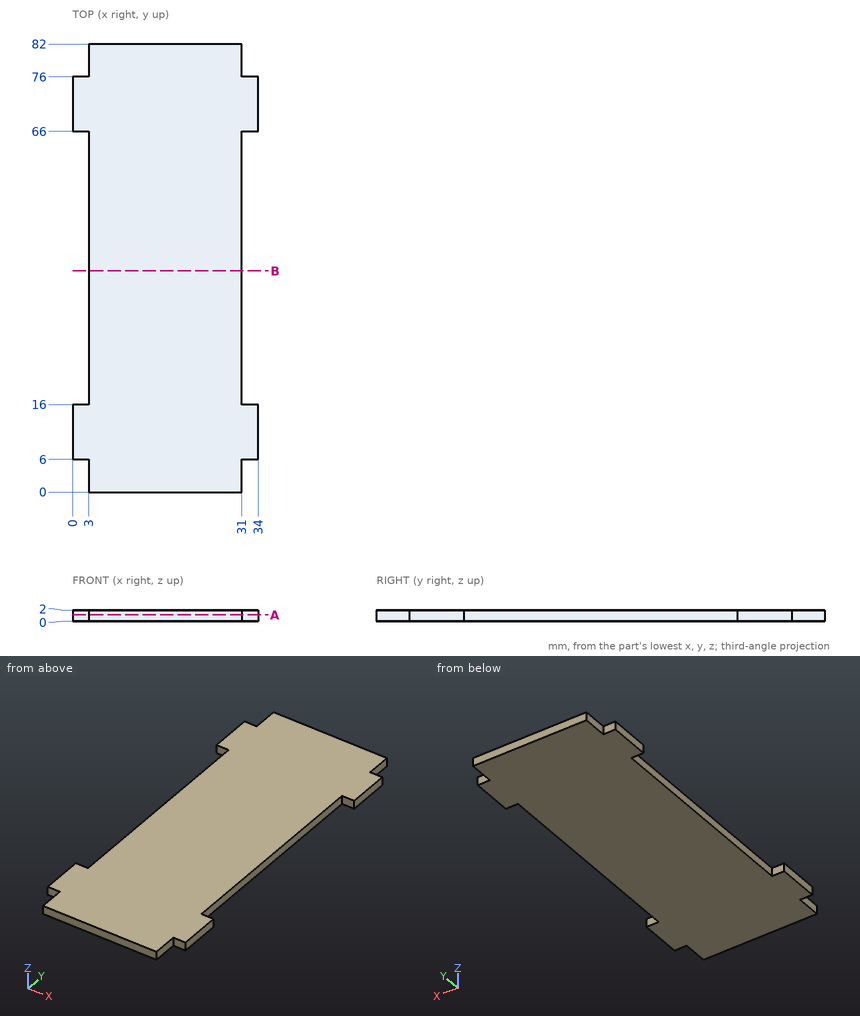
Geometry: see drawing. Coordinates: mm, zero at the bounding-box minimum. Give positions to 0.01 mm unless a question says otherwise; leave off trailing zeros. Order: outer loops, then holes, each group sorted by start corner. A loop starts at its lowest first (then second) coordinate and runs counter-clockwise, first axis right, second up. Notation, with made-up numbers: (-37, 88) - (3, 88) arc R15 ccw to (3, 117) - close; hole circle Ø2 at (25, 22). An arc over 180 degrees is marked (long way). Use a Markdown table: item, result.
(1) Section query A-A (z = 1.15). Output: boundary loops of the cut face in (x, y).
Computed values:
| item | result |
|---|---|
| outline | (0, 6) - (3, 6) - (3, 0) - (31, 0) - (31, 6) - (34, 6) - (34, 16) - (31, 16) - (31, 66) - (34, 66) - (34, 76) - (31, 76) - (31, 82) - (3, 82) - (3, 76) - (0, 76) - (0, 66) - (3, 66) - (3, 16) - (0, 16) - close |
(2) Section query B-B (y = 40.5). Output: boundary loops of the cut face in (x, z).
Computed values:
| item | result |
|---|---|
| outline | (3, 0) - (31, 0) - (31, 2) - (3, 2) - close |
(3) Line query: line 1 (Y direction, x = 2.5, z = 0.9); line 2 (X direction, y = 34.5, z = 0.7). Output: solid intervals per line, ascending. Write a range as from..to.
Computed values:
| item | result |
|---|---|
| line 1 | y = 6..16, 66..76 |
| line 2 | x = 3..31 |
(4) Pin query (flat end, axial travel): pin 1 (0.6 mm diameter, centred on y = 3, z = 1, fed in from +X); pin 2 (0.6 mm diameter, centred on y = 45.5, z = 1.5, fed in from -X); pin 3 (1 mm diameter, centred on x = 32, z = 0.5, fed in from -Y). Return the tip coordinate at first contact, or that it passes through.
Computed values:
| item | result |
|---|---|
| pin 1 | stops at x = 31 |
| pin 2 | stops at x = 3 |
| pin 3 | stops at y = 6 |
